```python
from build123d import *

# Parameters (mm, degrees)
SKETCH1_R                   = 650
BOSS_EXTRUDE1_DEPTH         = 60
SKETCH2_R                   = 205.5
CUT_EXTRUDE1_DEPTH          = 10
SKETCH3_R                   = 4
CUT_EXTRUDE2_DEPTH          = 25
M12_TAPPED_HOLE1_AT_2_COUNT = 2
M12_TAPPED_HOLE1_AT_2_PITCH = 311.769145362
M12_TAPPED_HOLE1_AT_3_COUNT = 2
M12_TAPPED_HOLE1_AT_3_PITCH = 311.769145362
CIRPATTERN1_COUNT           = 4
FILLET1_R                   = 1
SKETCH10_R                  = 5
CUT_EXTRUDE4_DEPTH          = 61
SKETCH11_R                  = 4.5
CUT_EXTRUDE5_DEPTH          = 61
SKETCH12_R                  = 9
CUT_EXTRUDE6_DEPTH          = 8.8
SKETCH14_R                  = 90
CUT_EXTRUDE8_DEPTH          = 7
CUT_EXTRUDE9_DEPTH          = 25


with BuildPart() as part:
    # Sketch1 → Boss-Extrude1 (new body)
    with BuildSketch(Plane(origin=(0, 0, 0), x_dir=(1, 0, 0), z_dir=(0, 1, 0))):
        Circle(SKETCH1_R)
    extrude(amount=-BOSS_EXTRUDE1_DEPTH)

    # Sketch2 → Cut-Extrude1 (cut)
    with BuildSketch(Plane(origin=(0, 0, 0), x_dir=(1, 0, 0), z_dir=(0, 1, 0))):
        with Locations((0, 400)):
            Circle(SKETCH2_R)
        with Locations((400, 0)):
            Circle(SKETCH2_R)
        with Locations((0, -400)):
            Circle(SKETCH2_R)
        with Locations((-400, 0)):
            Circle(SKETCH2_R)
    extrude(amount=-CUT_EXTRUDE1_DEPTH, mode=Mode.SUBTRACT)

    # Sketch3 → Cut-Extrude2 (cut)
    with BuildSketch(Plane(origin=(0, -10, 0), x_dir=(1, 0, 0), z_dir=(0, 1, 0))):
        with Locations((0, 575)):
            Circle(SKETCH3_R)
        with Locations((0, 225)):
            Circle(SKETCH3_R)
    cut_extrude2 = extrude(amount=-CUT_EXTRUDE2_DEPTH, mode=Mode.SUBTRACT)

    # Sketch9 → M12 Tapped Hole1 (revolve, cut)
    with BuildSketch(Plane(origin=(180, -10, -400), x_dir=(0, 0, 1), z_dir=(1, 0, 0))):
        Polygon((0, 0), (0, 29.25), (5.1, 26.185610843), (5.1, 0), align=None)
    m12_tapped_hole1 = revolve(axis=Axis((180, -3.65, -400), (0, -1, 0)), mode=Mode.SUBTRACT)

    # M12 Tapped Hole1 at 2: M12 Tapped Hole1 ×2
    with Locations(*[Vector(-0.866025404, 0, -0.5) * (i * M12_TAPPED_HOLE1_AT_2_PITCH) for i in range(1, M12_TAPPED_HOLE1_AT_2_COUNT)]):
        add(m12_tapped_hole1, mode=Mode.SUBTRACT)

    # M12 Tapped Hole1 at 3: M12 Tapped Hole1 ×2
    with Locations(*[Vector(-0.866025404, 0, 0.5) * (i * M12_TAPPED_HOLE1_AT_3_PITCH) for i in range(1, M12_TAPPED_HOLE1_AT_3_COUNT)]):
        add(m12_tapped_hole1, mode=Mode.SUBTRACT)

    # CirPattern1: M12 Tapped Hole1, Cut-Extrude2 ×4 about axis
    cirpattern1_axis = Axis((0, 0, 0), (0, 1, 0))
    for i in range(1, CIRPATTERN1_COUNT):
        add(m12_tapped_hole1.rotate(cirpattern1_axis, i * 360 / CIRPATTERN1_COUNT), mode=Mode.SUBTRACT)
        add(cut_extrude2.rotate(cirpattern1_axis, i * 360 / CIRPATTERN1_COUNT), mode=Mode.SUBTRACT)

    # CirPattern1 copy 1 sketch → CirPattern1 copy 1 (revolve, cut)
    with BuildSketch(Plane(origin=(-555.884572681, -10, 90), x_dir=(1, 0, 0), z_dir=(0, 0, -1))):
        Polygon((0, 0), (0, 29.25), (5.1, 26.185610843), (5.1, 0), align=None)
    revolve(axis=Axis((-555.884572681, -3.65, 90), (0, -1, 0)), mode=Mode.SUBTRACT)

    # CirPattern1 copy 2 sketch → CirPattern1 copy 2 (revolve, cut)
    with BuildSketch(Plane(origin=(90, -10, 555.884572681), x_dir=(0, 0, -1), z_dir=(-1, 0, 0))):
        Polygon((0, 0), (0, 29.25), (5.1, 26.185610843), (5.1, 0), align=None)
    revolve(axis=Axis((90, -3.65, 555.884572681), (0, -1, 0)), mode=Mode.SUBTRACT)

    # CirPattern1 copy 3 sketch → CirPattern1 copy 3 (revolve, cut)
    with BuildSketch(Plane(origin=(555.884572681, -10, -90), x_dir=(-1, 0, 0), z_dir=(0, 0, 1))):
        Polygon((0, 0), (0, 29.25), (5.1, 26.185610843), (5.1, 0), align=None)
    revolve(axis=Axis((555.884572681, -3.65, -90), (0, -1, 0)), mode=Mode.SUBTRACT)

    # CirPattern1 copy 4 sketch → CirPattern1 copy 4 (revolve, cut)
    with BuildSketch(Plane(origin=(-244.115427319, -10, 90), x_dir=(1, 0, 0), z_dir=(0, 0, -1))):
        Polygon((0, 0), (0, 29.25), (5.1, 26.185610843), (5.1, 0), align=None)
    revolve(axis=Axis((-244.115427319, -3.65, 90), (0, -1, 0)), mode=Mode.SUBTRACT)

    # CirPattern1 copy 5 sketch → CirPattern1 copy 5 (revolve, cut)
    with BuildSketch(Plane(origin=(90, -10, 244.115427319), x_dir=(0, 0, -1), z_dir=(-1, 0, 0))):
        Polygon((0, 0), (0, 29.25), (5.1, 26.185610843), (5.1, 0), align=None)
    revolve(axis=Axis((90, -3.65, 244.115427319), (0, -1, 0)), mode=Mode.SUBTRACT)

    # CirPattern1 copy 6 sketch → CirPattern1 copy 6 (revolve, cut)
    with BuildSketch(Plane(origin=(244.115427319, -10, -90), x_dir=(-1, 0, 0), z_dir=(0, 0, 1))):
        Polygon((0, 0), (0, 29.25), (5.1, 26.185610843), (5.1, 0), align=None)
    revolve(axis=Axis((244.115427319, -3.65, -90), (0, -1, 0)), mode=Mode.SUBTRACT)

    # Fillet1
    fillet1_edges = [part.edges().sort_by_distance(p)[0] for p in [
        (-650, 0, 0),
        (-650, -60, 0),
    ]]
    fillet(fillet1_edges, radius=FILLET1_R)

    # Sketch10 → Cut-Extrude4 (cut, through all)
    with BuildSketch(Plane(origin=(0, 0, 0), x_dir=(1, 0, 0), z_dir=(0, 1, 0))):
        with Locations((0, 110)):
            Circle(SKETCH10_R)
        with Locations((0, -110)):
            Circle(SKETCH10_R)
    extrude(amount=-CUT_EXTRUDE4_DEPTH, mode=Mode.SUBTRACT)

    # Sketch11 → Cut-Extrude5 (cut, through all)
    with BuildSketch(Plane(origin=(0, 0, 0), x_dir=(1, 0, 0), z_dir=(0, 1, 0))):
        with Locations((101.626748576, 42.09517756)):
            Circle(SKETCH11_R)
        with Locations((101.626748576, -42.09517756)):
            Circle(SKETCH11_R)
        with Locations((42.09517756, 101.626748576)):
            Circle(SKETCH11_R)
        with Locations((42.09517756, -101.626748576)):
            Circle(SKETCH11_R)
        with Locations((-42.09517756, 101.626748576)):
            Circle(SKETCH11_R)
        with Locations((-42.09517756, -101.626748576)):
            Circle(SKETCH11_R)
        with Locations((-101.626748576, 42.09517756)):
            Circle(SKETCH11_R)
        with Locations((-101.626748576, -42.09517756)):
            Circle(SKETCH11_R)
    extrude(amount=-CUT_EXTRUDE5_DEPTH, mode=Mode.SUBTRACT)

    # Sketch12 → Cut-Extrude6 (cut)
    with BuildSketch(Plane(origin=(0, 0, 0), x_dir=(1, 0, 0), z_dir=(0, 1, 0))):
        with Locations((-42.09517756, 101.626748576)):
            Circle(SKETCH12_R)
        with Locations((42.09517756, 101.626748576)):
            Circle(SKETCH12_R)
        with Locations((101.626748576, 42.09517756)):
            Circle(SKETCH12_R)
        with Locations((101.626748576, -42.09517756)):
            Circle(SKETCH12_R)
        with Locations((42.09517756, -101.626748576)):
            Circle(SKETCH12_R)
        with Locations((-42.09517756, -101.626748576)):
            Circle(SKETCH12_R)
        with Locations((-101.626748576, -42.09517756)):
            Circle(SKETCH12_R)
        with Locations((-101.626748576, 42.09517756)):
            Circle(SKETCH12_R)
    extrude(amount=-CUT_EXTRUDE6_DEPTH, mode=Mode.SUBTRACT)

    # Sketch14 → Cut-Extrude8 (cut)
    with BuildSketch(Plane.XZ.offset(60)):
        Circle(SKETCH14_R)
    extrude(amount=-CUT_EXTRUDE8_DEPTH, mode=Mode.SUBTRACT)

    # Sketch15 → Cut-Extrude9 (cut)
    with BuildSketch(Plane(origin=(0, 0, 0), x_dir=(1, 0, 0), z_dir=(0, 1, 0))):
        with BuildLine():
            Line((0, -14.142135624), (-7.071067812, -7.071067812))
            Line((-7.071067812, -7.071067812), (-14.142135624, 0))
            Line((-14.142135624, 0), (-465.928888929, -451.786753305))
            ThreePointArc((-465.928888929, -451.786753305), (-458.91230099, -458.91230099), (-451.786753305, -465.928888929))
            Line((-451.786753305, -465.928888929), (0, -14.142135624))
        make_face()
        with BuildLine():
            Line((465.928888929, -451.786753305), (14.142135624, 0))
            Line((14.142135624, 0), (7.071067812, -7.071067812))
            Line((7.071067812, -7.071067812), (0, -14.142135624))
            Line((0, -14.142135624), (451.786753305, -465.928888929))
            ThreePointArc((451.786753305, -465.928888929), (458.91230099, -458.91230099), (465.928888929, -451.786753305))
        make_face()
        with BuildLine():
            Line((0, 14.142135624), (7.071067812, 7.071067812))
            Line((7.071067812, 7.071067812), (14.142135624, 0))
            Line((14.142135624, 0), (465.928888929, 451.786753305))
            ThreePointArc((465.928888929, 451.786753305), (458.91230099, 458.91230099), (451.786753305, 465.928888929))
            Line((451.786753305, 465.928888929), (0, 14.142135624))
        make_face()
        with BuildLine():
            Line((-7.071067812, 7.071067812), (0, 14.142135624))
            Line((0, 14.142135624), (-451.786753305, 465.928888929))
            ThreePointArc((-451.786753305, 465.928888929), (-458.91230099, 458.91230099), (-465.928888929, 451.786753305))
            Line((-465.928888929, 451.786753305), (-14.142135624, 0))
            Line((-14.142135624, 0), (-7.071067812, 7.071067812))
        make_face()
        Polygon((-7.071067812, -7.071067812), (0, 0), (-7.071067812, 7.071067812), (-14.142135624, 0), align=None)
        Polygon((7.071067812, -7.071067812), (0, 0), (-7.071067812, -7.071067812), (0, -14.142135624), align=None)
        Polygon((14.142135624, 0), (7.071067812, 7.071067812), (0, 0), (7.071067812, -7.071067812), align=None)
        Polygon((0, 0), (7.071067812, 7.071067812), (0, 14.142135624), (-7.071067812, 7.071067812), align=None)
        with BuildLine():
            ThreePointArc((-451.786753305, -465.928888929), (-458.91230099, -458.91230099), (-465.928888929, -451.786753305))
            Line((-465.928888929, -451.786753305), (-487.712976159, -473.570840535))
            Line((-487.712976159, -473.570840535), (-473.570840535, -487.712976159))
            Line((-473.570840535, -487.712976159), (-451.786753305, -465.928888929))
        make_face()
        with BuildLine():
            ThreePointArc((-465.928888929, 451.786753305), (-458.91230099, 458.91230099), (-451.786753305, 465.928888929))
            Line((-451.786753305, 465.928888929), (-461.131853897, 475.27398952))
            Line((-461.131853897, 475.27398952), (-475.27398952, 461.131853897))
            Line((-475.27398952, 461.131853897), (-465.928888929, 451.786753305))
        make_face()
        with BuildLine():
            Line((456.45101614, 470.593151764), (451.786753305, 465.928888929))
            ThreePointArc((451.786753305, 465.928888929), (458.91230099, 458.91230099), (465.928888929, 451.786753305))
            Line((465.928888929, 451.786753305), (470.593151764, 456.45101614))
            Line((470.593151764, 456.45101614), (456.45101614, 470.593151764))
        make_face()
        with BuildLine():
            Line((476.238577972, -462.096442349), (465.928888929, -451.786753305))
            ThreePointArc((465.928888929, -451.786753305), (458.91230099, -458.91230099), (451.786753305, -465.928888929))
            Line((451.786753305, -465.928888929), (462.096442349, -476.238577972))
            Line((462.096442349, -476.238577972), (476.238577972, -462.096442349))
        make_face()
    extrude(amount=-CUT_EXTRUDE9_DEPTH, mode=Mode.SUBTRACT)


solid = part.part
```
The listing builds one solid part. Answer for the finished solid, in the listing's coordinates (mm). A direction names the side the tool comes from. Round coordinates to 2 decimals unless told otherwise and drop trailing zeros. Use one line per item in the form item = value. Start each with the question number.
1. Given pin 1 Ø8 at (y, z) = (-41.5, -404.5) entering from -X; pin 2 Ø9 at (x, z) = (-244.12, 90) entering from +Y; pin 3 Ø13 at (x, z) = (225, 0) entering from +Y; pin 4 Ø6 at (x, z) = (0, 110) entering from +Y, each flat-ended and moving along its own axis, determine where each tip first touches the part or whether it passes through.
2. A tool of negligible diameter and unlimited length cuts with its end or side. For faces 4 (the face through (41.53, -56.549, -79.845)), 5 (the face through (-605.3, -4.93, -9.04)), 6 (the face through (-207, 0, 398)), from which of +Z, -Z, +X, -X, +Y, -Y can it reach the whole face along a straight path? Write none if from no direction.
3. For a pull along X with two mould halves and no side action, classify faces 1 (the face through (-44.548, -4.93, -199.387)), 2 (the face through (398, 0, -207)), 3 (the face through (619.984, -29.594, -195.242)) as pulls with the +X half, pulls with the -X half, needs draft (parallel to the pull), parting line crosses it, or undercut.
4. Consider line 1 (X direction, y = -15.5, z = 0); line 2 (Z direction, x = -84, y = -20.5); line 3 (Z direction, x = 113.5, y = -24.5). Determine where each line is inside the solid, lowest interval first. Write a range as [from, to].
Geometry check:
q1.pin_1 = -511.96
q1.pin_2 = -36.54
q1.pin_3 = -10
q1.pin_4 = through
q2.face_4 = -Y
q2.face_5 = +Y
q2.face_6 = +Z, -Z, +X, -X, +Y
q3.face_1 = undercut
q3.face_2 = needs draft
q3.face_3 = parting line crosses it
q4.line_1 = [-650, -579], [-571, -229], [-221, -14.14], [14.14, 221], [229, 571], [579, 650]
q4.line_2 = [-644.55, -98.14], [-69.86, 69.86], [98.14, 644.55]
q4.line_3 = [-640.01, -127.64], [-99.36, 99.36], [127.64, 640.01]
